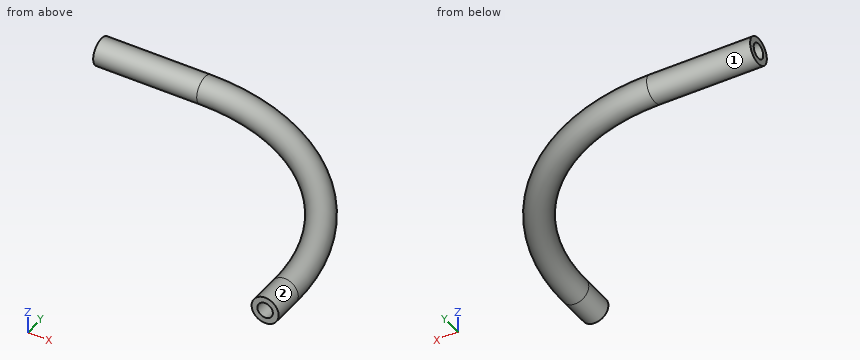
```python
from build123d import *

# Parameters (mm, degrees)
SKETCH2_R   = 8.5
SKETCH2_R_2 = 4.85


with BuildPart() as part:
    # Sweep1: sweep along a curve in space
    with BuildLine() as sweep1_path:
        Line((-63.953291268, 176.442341084, 4.917581679), (1.046708732, 176.442341084, 4.917581679))
        ThreePointArc((1.046708732, 176.442341084, 4.917581679), (93.239290863, 138.254923215, 4.917581679), (131.426708732, 46.062341084, 4.917581679))
        Line((131.426708732, 26.062341084, 4.917581679), (131.426708732, 46.062341084, 4.917581679))
    # Sketch2 → Sweep1 (sweep)
    with BuildSketch(Plane(origin=(-63.953291268, 176.442341084, 4.917581679), x_dir=(0, 0, -1), z_dir=(1, 0, 0))):
        Circle(SKETCH2_R)
        Circle(SKETCH2_R_2, mode=Mode.SUBTRACT)
    sweep(path=sweep1_path.line)


solid = part.part
```
Part model, mm, in its own coordinate system. Face numbers are marked on the shaded views. A direction names the side the tool comes from. Round coordinates to 2 decimals unless told otherwise and drop trailing zeros. Order: outer loops, then holes, each group sorted by start corner. A loop starts at its lowest first (then second) coordinate and runs counter-clockwise, first axis right, second up. Notation, with made-up numbers: M 72.5,72.25 L 103.5,72.25 A20 ccw 103.5,106.25 Z; hole C 82,-1 d11. An arc over 180 degrees is marked long. Answer in a Markdown table with one row per item. Add a question column.
Q1. Cut at A-A on z = 7. Give the cut face in (x, y), and give its area (3 significant figures).
Q2. Wall check: L1, parallel to Y at x = -26, z = 4.5; L2, parallel to Y at x = -12, z = 9; L3, parallel to X at y = 64, z = 6.5. Give the ranges that are in metal, low to high. Write a range as from..to.
Q3. 3-axis set-ups, long thin cutter, end or side, ignore diameter. For the marked faces 1 and 2: which of +Z, -Z, +X, -X, +Y, -Y reach the whole face in a straight line?
Q4. Pin check, flat tips, straight feed: pin 1 (8.5 mm diameter, centred on y = 176.44, z = 4.92, fed in from +X); pin 2 (10 mm diameter, centred on x = 43.5, z = 2, fed in from +Y); pin 3 (10 mm diameter, centred on y = 136, z = -0.5, fed in from -X). Stop position of each tip, or through.
Q5. Cut at B-B on x = -44.5. Give the cut face in (y, z), and give its area (3 significant figures).
Established:
| question | item | result |
|---|---|---|
| 1 | outline | M -63.95,168.2 L 1.05,168.2 A122.14 cw 123.19,46.06 L 123.19,26.06 L 127.05,26.06 L 127.05,46.06 A126 ccw 1.05,172.06 L -63.95,172.06 Z; M -63.95,180.82 L 1.05,180.82 A134.76 cw 135.81,46.06 L 135.81,26.06 L 139.67,26.06 L 139.67,46.06 A138.62 ccw 1.05,184.68 L -63.95,184.68 Z |
| 1 | area | 2,240 mm2 |
| 2 | L1 | y = 167.95..171.61, 181.27..184.93 |
| 2 | L2 | y = 168.99..173.82, 179.06..183.9 |
| 2 | L3 | x = 121.75..125.56, 134.81..138.61 |
| 3 | face 1 | -X |
| 3 | face 2 | -Y |
| 4 | pin 1 | stops at x = 59.18 |
| 4 | pin 2 | stops at y = 179.63 |
| 4 | pin 3 | stops at x = 79.1 |
| 5 | outline | C 176.44,4.92 d17; hole C 176.44,4.92 d9.7 |
| 5 | area | 153 mm2 |
